```python
from build123d import *

# Parameters (mm, degrees)
SK_DISCO_R           = 29.572962734
DISCO_DEPTH          = 1.8
HUECO_DIENTE_DEPTH   = 42.861202201
MATRIZ_DIENTES_COUNT = 13


with BuildPart() as part:
    # Sk_Disco → Disco (new body)
    with BuildSketch(Plane.XY):
        Circle(SK_DISCO_R)
        with BuildLine():
            Line((2.6, 17.305779381), (2.6, 16.293863876))
            ThreePointArc((2.6, 16.293863876), (0, 16.5), (-2.6, 16.293863876))
            Line((-2.6, 16.293863876), (-2.6, 17.305779381))
            ThreePointArc((-2.6, 17.305779381), (-6.362648192, 16.302352836), (-9.810241185, 14.491693065))
            Line((-9.810241185, 14.491693065), (-9.163816615, 13.721314261))
            ThreePointArc((-9.163816615, 13.721314261), (-10.60599556, 12.639733311), (-11.92157661, 11.407278866))
            Line((-11.92157661, 11.407278866), (-12.56800118, 12.17765767))
            ThreePointArc((-12.56800118, 12.17765767), (-15.155444566, 8.75), (-16.830161491, 4.795379462))
            Line((-16.830161491, 4.795379462), (-15.839781591, 4.620748764))
            ThreePointArc((-15.839781591, 4.620748764), (-16.249327925, 2.865194932), (-16.464915031, 1.075440854))
            Line((-16.464915031, 1.075440854), (-17.455294931, 1.250071551))
            ThreePointArc((-17.455294931, 1.250071551), (-17.234135678, -3.038843109), (-15.975062189, -7.144745486))
            Line((-15.975062189, -7.144745486), (-15.104136721, -6.641916433))
            ThreePointArc((-15.104136721, -6.641916433), (-14.289419162, -8.25), (-13.304136721, -9.759607887))
            Line((-13.304136721, -9.759607887), (-14.175062189, -10.26243694))
            ThreePointArc((-14.175062189, -10.26243694), (-11.24878317, -13.405777755), (-7.645053746, -15.741764616))
            Line((-7.645053746, -15.741764616), (-7.301098416, -14.796755115))
            ThreePointArc((-7.301098416, -14.796755115), (-5.643332365, -15.504928243), (-3.918204981, -16.028027631))
            Line((-3.918204981, -16.028027631), (-4.262160311, -16.973037132))
            ThreePointArc((-4.262160311, -16.973037132), (0, -17.5), (4.262160311, -16.973037132))
            Line((4.262160311, -16.973037132), (3.918204981, -16.028027631))
            ThreePointArc((3.918204981, -16.028027631), (5.643332365, -15.504928243), (7.301098416, -14.796755115))
            Line((7.301098416, -14.796755115), (7.645053746, -15.741764616))
            ThreePointArc((7.645053746, -15.741764616), (11.24878317, -13.405777755), (14.175062189, -10.26243694))
            Line((14.175062189, -10.26243694), (13.304136721, -9.759607887))
            ThreePointArc((13.304136721, -9.759607887), (14.289419162, -8.25), (15.104136721, -6.641916433))
            Line((15.104136721, -6.641916433), (15.975062189, -7.144745486))
            ThreePointArc((15.975062189, -7.144745486), (17.234135678, -3.038843109), (17.455294931, 1.250071551))
            Line((17.455294931, 1.250071551), (16.464915031, 1.075440854))
            ThreePointArc((16.464915031, 1.075440854), (16.249327925, 2.865194932), (15.839781591, 4.620748764))
            Line((15.839781591, 4.620748764), (16.830161491, 4.795379462))
            ThreePointArc((16.830161491, 4.795379462), (15.155444566, 8.75), (12.56800118, 12.17765767))
            Line((12.56800118, 12.17765767), (11.92157661, 11.407278866))
            ThreePointArc((11.92157661, 11.407278866), (10.60599556, 12.639733311), (9.163816615, 13.721314261))
            Line((9.163816615, 13.721314261), (9.810241185, 14.491693065))
            ThreePointArc((9.810241185, 14.491693065), (6.362648192, 16.302352836), (2.6, 17.305779381))
        make_face(mode=Mode.SUBTRACT)
    extrude(amount=DISCO_DEPTH)

    # Sk_Hueco → Hueco_diente (cut, through all)
    with BuildSketch(Plane.XY):
        with BuildLine():
            ThreePointArc((-3.859493724, 25.582712562), (0, 22.558992327), (3.859493724, 25.582712562))
            ThreePointArc((3.859493724, 25.582712562), (5.159504407, 28.464173723), (7.400896702, 30.693300634))
            ThreePointArc((7.400896702, 30.693300634), (0, 31.572962734), (-7.400896702, 30.693300634))
            ThreePointArc((-7.400896702, 30.693300634), (-5.159504407, 28.464173723), (-3.859493724, 25.582712562))
        make_face()
    hueco_diente = extrude(amount=HUECO_DIENTE_DEPTH, mode=Mode.SUBTRACT)

    # Matriz_dientes: Hueco_diente ×13 about axis
    matriz_dientes_axis = Axis((0, 0, 0), (0, 0, 1))
    for i in range(1, MATRIZ_DIENTES_COUNT):
        add(hueco_diente.rotate(matriz_dientes_axis, i * 360 / MATRIZ_DIENTES_COUNT), mode=Mode.SUBTRACT)


solid = part.part
```
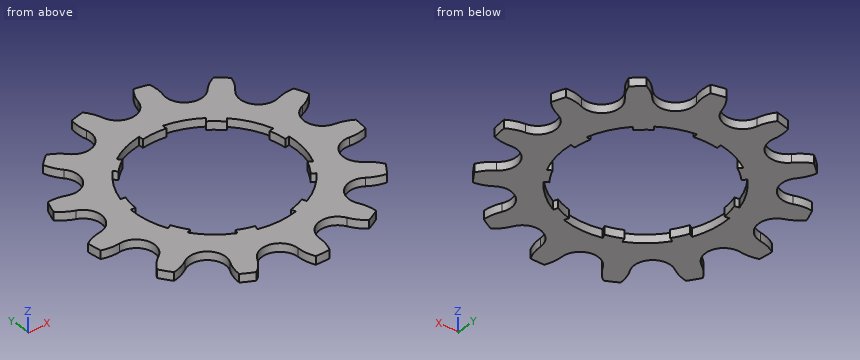
Read the model definition and answer for the solid it produces. Units are mm, in the model's axes. Coordinates: 2 decimals unless noted, no trailing zeros. Order: outer loops, then holes, each group sorted by start corner. A loop starts at its lowest first (then second) coordinate and runs counter-clockwise, first axis right, second up. Notation, with made-up numbers: (-2, 27.5) - (45, 27.5) arc R17 cw to (45, 41.5) - close; hole circle Ø11 at (18.5, -31). An arc over 180 degrees is marked (long way). Answer as a JSON object with one key per item and string values. Group by question number.
Item 1: Section A-A (y = -11) is taken. Give the vertices of the cut face in (x, z), plus the area to 3 significant figures.
Item 2: A flat-ended cylindrical pin translates along its axis: P1, Ø1, axis at y = -5.5, z = 1, coming from the -X side. Find the tip coordinate at first contact, or state that the pin passes through.
Item 3: Consider probe 1 along X at (y, z) = (12, 1.2); probe 2 along X at (y, z) = (-25, 0.5); probe 3 along X at (y, z) = (-24.5, 1.5). Determine where each line is inside the solid, lowest interval first. Write a range as from..to.
Results are:
{
 "1": {"outline": "(-21.17, 0) - (-13.61, 0) - (-13.61, 1.8) - (-21.17, 1.8) - close; (13.61, 0) - (21.17, 0) - (21.17, 1.8) - (13.61, 1.8) - close", "area": "27.2 mm^2"},
 "2": {"P1": "stops at x = -29.15"},
 "3": {"probe 1": "x = -19.32..-12.74, -12.42..-11.32, 11.32..12.42, 12.74..19.32", "probe 2": "x = -15.04..-10.54, -2.45..2.45, 10.54..15.04", "probe 3": "x = -14.98..-10.21, -2.58..2.58, 10.21..14.98"}
}
